Geometry check sheet. Reference: the model listing, model coordinates, mm. Face numbers are marked on the shaded views. Round coordinates to 2 decimals unless told otherwise and drop trailing zeros. Order: outer loops, then holes, each group sorted by start corner. A loop starts at its lowest first (then second) coordinate and runs counter-clockwise, first axis right, second up. Notation, with made-up numbers: (2, 87) - (10, 87) arc R28 ccw to (10, 120) - close; hole circle Ø2 at (18, -10.75). An arc over 180 degrees is marked (long way). Write each question's results on one line, items separated by ' | '.
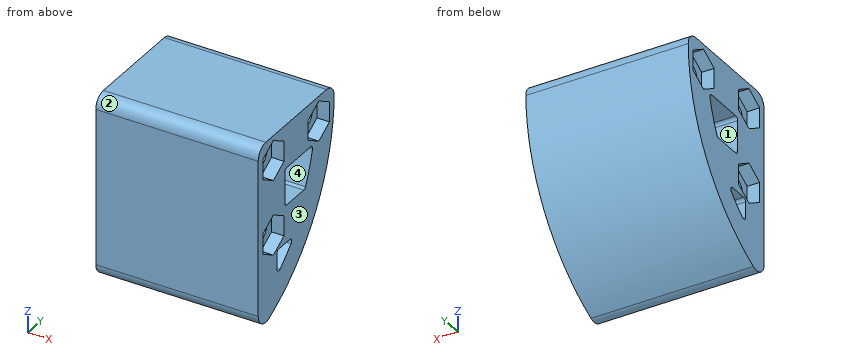
```python
from build123d import *

# Parameters (mm, degrees)
SKETCH1_R           = 1.5
BOSS_EXTRUDE1_DEPTH = 26
CUT_EXTRUDE1_DEPTH  = 2
CUT_EXTRUDE2_START  = 26
CUT_EXTRUDE2_DEPTH  = 2


with BuildPart() as part:
    # Sketch1 → Boss-Extrude1 (new body)
    with BuildSketch(Plane(origin=(0, 0, 0), x_dir=(0, 0, -1), z_dir=(1, 0, 0))):
        with BuildLine():
            Line((-4, 14.045215535), (-4, -2))
            ThreePointArc((-4, -2), (-3.414213562, -3.414213562), (-2, -4))
            Line((-2, -4), (23, -4))
            ThreePointArc((23, -4), (24.68931411, -3.070615635), (24.808606098, -1.146217837))
            ThreePointArc((24.808606098, -1.146217837), (13.883506503, 11.294438637), (-1.977108188, 16.045084522))
            ThreePointArc((-1.977108188, 16.045084522), (-3.406096792, 15.467499547), (-4, 14.045215535))
        make_face()
        Circle(SKETCH1_R, mode=Mode.SUBTRACT)
        with Locations((0, 12)):
            Circle(SKETCH1_R, mode=Mode.SUBTRACT)
        with Locations((12, 0)):
            Circle(SKETCH1_R, mode=Mode.SUBTRACT)
        with BuildLine():
            Line((3, 9.845620053), (3, 3.5))
            ThreePointArc((3, 3.5), (3.146446609, 3.146446609), (3.5, 3))
            Line((3.5, 3), (8.5, 3))
            ThreePointArc((8.5, 3), (8.853553391, 3.146446609), (9, 3.5))
            Line((9, 3.5), (9, 8.028111937))
            ThreePointArc((9, 8.028111937), (8.92450743, 8.292296422), (8.720826232, 8.476705043))
            ThreePointArc((8.720826232, 8.476705043), (6.220295037, 9.542901904), (3.618785416, 10.331305162))
            ThreePointArc((3.618785416, 10.331305162), (3.191287114, 10.238934627), (3, 9.845620053))
        make_face(mode=Mode.SUBTRACT)
        with BuildLine():
            Line((15, 4.286575508), (15, 1.427805862))
            ThreePointArc((15, 1.427805862), (15.146446609, 1.074252472), (15.5, 0.927805862))
            Line((15.5, 0.927805862), (18.01869702, 0.927805862))
            ThreePointArc((18.01869702, 0.927805862), (18.466352985, 1.205086001), (18.417504517, 1.729389316))
            ThreePointArc((18.417504517, 1.729389316), (17.187978253, 3.234831626), (15.849421282, 4.644213269))
            ThreePointArc((15.849421282, 4.644213269), (15.305977631, 4.747395777), (15, 4.286575508))
        make_face(mode=Mode.SUBTRACT)
    extrude(amount=BOSS_EXTRUDE1_DEPTH)

    # Sketch2 → Cut-Extrude1 (cut)
    with BuildSketch(Plane(origin=(0, 0, 0), x_dir=(0, 0, -1), z_dir=(1, 0, 0))):
        Polygon((-1.616580754, 9.2), (1.616580754, 9.2), (3.233161507, 12), (1.616580754, 14.8), (-1.616580754, 14.8), (-3.233161507, 12), align=None)
        Polygon((1.616580754, 2.8), (-1.616580754, 2.8), (-3.233161507, 0), (-1.616580754, -2.8), (1.616580754, -2.8), (3.233161507, 0), align=None)
        Polygon((15.233161507, 0), (13.616580754, 2.8), (10.383419246, 2.8), (8.766838493, 0), (10.383419246, -2.8), (13.616580754, -2.8), align=None)
    extrude(amount=CUT_EXTRUDE1_DEPTH, mode=Mode.SUBTRACT)

    # Sketch2<3> → Cut-Extrude2 (cut)
    with BuildSketch(Plane(origin=(0, 0, 0), x_dir=(0, 0, -1), z_dir=(1, 0, 0)).offset(CUT_EXTRUDE2_START)):
        Polygon((-1.616580754, 9.2), (1.616580754, 9.2), (3.233161507, 12), (1.616580754, 14.8), (-1.616580754, 14.8), (-3.233161507, 12), align=None)
        Polygon((1.616580754, 2.8), (-1.616580754, 2.8), (-3.233161507, 0), (-1.616580754, -2.8), (1.616580754, -2.8), (3.233161507, 0), align=None)
        Polygon((15.233161507, 0), (13.616580754, 2.8), (10.383419246, 2.8), (8.766838493, 0), (10.383419246, -2.8), (13.616580754, -2.8), align=None)
    extrude(amount=-CUT_EXTRUDE2_DEPTH, mode=Mode.SUBTRACT)


solid = part.part
```
(1) Section check A-A (y = 6). Record the cut outline in (x, z), then the cut area to 3 significant figures.
Answers follow:
outline: (0, -20.08) - (26, -20.08) - (26, -9) - (0, -9) - close; (0, -3) - (26, -3) - (26, 4) - (0, 4) - close | area: 470 mm²
(2) Material ranges on line 1 (Z direction, x = 16.25, y = 6); line 2 (Z direction, x = 13.25, y = 12.75); line 3 (Z direction, x = 16, y = 0), recorded low to high.
Answers follow:
line 1: -20.08 to -9, -3 to 4 | line 2: -11.35 to -1.3, 1.3 to 4 | line 3: -24.24 to -13.5, -10.5 to -1.5, 1.5 to 4
(3) Section check D-D (y = 0.5). Record the cut outline in (x, z).
Answers follow:
outline: (0, -23.97) - (26, -23.97) - (26, -14.94) - (24, -14.94) - (24, -13.41) - (2, -13.41) - (2, -14.94) - (0, -14.94) - close; (0, -9.06) - (2, -9.06) - (2, -10.59) - (24, -10.59) - (24, -9.06) - (26, -9.06) - (26, -2.94) - (24, -2.94) - (24, -1.41) - (2, -1.41) - (2, -2.94) - (0, -2.94) - close; (0, 2.94) - (2, 2.94) - (2, 1.41) - (24, 1.41) - (24, 2.94) - (26, 2.94) - (26, 4) - (0, 4) - close
(4) Draft check along Y on the marked faces 1, 2, 3 and 4. Enter one of: released by +Y, released by -Y, zero draft, split by the parting line, or undercut.
Answers follow:
face 1: undercut | face 2: released by -Y | face 3: zero draft | face 4: undercut
(5) Section check C-C (x = 6.75). Record the cut outline in (y, z), then the cut area to 3 significant figures.
Answers follow:
outline: (-4, -23) arc R2 ccw to (-1.15, -24.81) arc R30 ccw to (16.05, 1.98) arc R2 ccw to (14.05, 4) - (-2, 4) arc R2 ccw to (-4, 2) - close; hole circle Ø3 at (0, -12); hole circle Ø3 at (0, 0); hole (0.93, -18.02) arc R0.5 ccw to (1.73, -18.42) arc R26 ccw to (4.64, -15.85) arc R0.5 ccw to (4.29, -15) - (1.43, -15) arc R0.5 ccw to (0.93, -15.5) - close; hole (3, -8.5) arc R0.5 ccw to (3.5, -9) - (8.03, -9) arc R0.5 ccw to (8.48, -8.72) arc R25 ccw to (10.33, -3.62) arc R0.5 ccw to (9.85, -3) - (3.5, -3) arc R0.5 ccw to (3, -3.5) - close; hole circle Ø3 at (12, 0) | area: 374 mm²
(6) Depth check by flat-ended pin: pin 1 Ø5 at (x, y) = (16, 1.5) entering from -Z; pin 2 Ø1 at (x, z) = (25, -12.5) entering from +Y; pin 3 Ø4 at (x, z) = (15.5, -15.5) entering from +Y. Enter the tip coordinate at first touch or a pass-through.
Answers follow:
pin 1: z = -24.74 | pin 2: y = 12.41 | pin 3: y = 11.54
(7) Section check B-B (z = -12). Record the cut outline in (x, y).
Answers follow:
outline: (0, -4) - (26, -4) - (26, -2.8) - (24, -2.8) - (24, -1.5) - (2, -1.5) - (2, -2.8) - (0, -2.8) - close; (0, 2.8) - (2, 2.8) - (2, 1.5) - (24, 1.5) - (24, 2.8) - (26, 2.8) - (26, 12.41) - (0, 12.41) - close
